Source: CAD feature listing. Evaluate the final solid. Frame: model axes, mm. A direction names the side the tool comes from. Give positions to 0.01 mm unless a question says otherwise; leave off trailing zeros. Write each loop counter-clockwise with the first axis right and the second up, starting at its lowest first coordinate (ties: lowest second). Pieces come first, ordered by that corner, then holes. Notation, with made-up numbers: (80.5, 61.25) -> (106.5, 61.25) arc R22 cw to (106.5, 84.25) -> close; hole circle Ø2 at (4, 88). An arc over 180 degrees is marked (long way). Use a Markdown table: item, result. Add a question column.
```python
from build123d import *

# Parameters (mm, degrees)
F0_W      = 51
F0_H      = 26
F1_DEPTH  = 1.5
F2_W      = 2
F2_H      = 2
F3_DEPTH  = 13
F5_DEPTH  = 13
F6_W      = 4
F6_H      = 2.5
F7_DEPTH  = 2.5
F8_R      = 0.75
F9_DEPTH  = 1.501
F11_DEPTH = 2
F12_W     = 8
F12_H     = 5
F13_DEPTH = 1.2


with BuildPart() as f1:
    # F0 (on Top) → F1 (new body)
    with BuildSketch(Plane.XY):
        Rectangle(F0_W, F0_H)
    extrude(amount=F1_DEPTH)

    # F2 (on face) → F3 (join)
    with BuildSketch(Plane.XY.offset(1.5)):
        with Locations((-24.5, 8.4)):
            Rectangle(F2_W, F2_H)
        Polygon((-19.5, 11.4), (-25.5, 11.4), (-25.5, 9.4), (-23.5, 9.4), (-21.5, 9.4), (-19.5, 9.4), align=None)
        with Locations((-20.5, 8.4)):
            Rectangle(F2_W, F2_H)
        with Locations((-24.5, -8.4)):
            Rectangle(F2_W, F2_H)
        Polygon((-23.5, -9.4), (-25.5, -9.4), (-25.5, -11.4), (-19.5, -11.4), (-19.5, -9.4), (-21.5, -9.4), align=None)
        with Locations((-20.5, -8.4)):
            Rectangle(F2_W, F2_H)
    extrude(amount=F3_DEPTH)

    # F4 (on face) → F5 (join)
    with BuildSketch(Plane.XY.offset(1.5)):
        Polygon((-19.5, 10.5), (-19.5, 9.15), (24.3, 9.15), (24.3, -9.15), (-19.5, -9.15), (-19.5, -10.5), (25.5, -10.5), (25.5, 10.5), align=None)
    extrude(amount=F5_DEPTH)

    # F6 (on face) → F7 (join)
    with BuildSketch(Plane.XY.offset(1.5)):
        Polygon((-15.5, 9.15), (-19.5, 9.15), (-19.5, 7.4), (-19.5, 6.65), (-15.5, 6.65), align=None)
        with Locations((22.3, 7.9)):
            Rectangle(F6_W, F6_H)
        with Locations((22.3, -7.9)):
            Rectangle(F6_W, F6_H)
        Polygon((-19.5, -9.15), (-15.5, -9.15), (-15.5, -6.65), (-19.5, -6.65), (-19.5, -7.4), align=None)
    extrude(amount=F7_DEPTH)

    # F8 (on face) → F9 (cut, through all)
    with BuildSketch(Plane.XY.offset(1.5)):
        with Locations((-18.5, 11.5)):
            Circle(F8_R)
        with Locations((2.5, 11.5)):
            Circle(F8_R)
        with Locations((23.5, 11.5)):
            Circle(F8_R)
        with Locations((-18.5, -11.5)):
            Circle(F8_R)
        with Locations((2.5, -11.5)):
            Circle(F8_R)
        with Locations((23.5, -11.5)):
            Circle(F8_R)
    extrude(amount=-F9_DEPTH, mode=Mode.SUBTRACT)

    # F10 (on face) → F11 (cut)
    with BuildSketch(Plane.XY.offset(1.5)):
        Polygon((-21.5, 9.4), (-23.5, 9.4), (-23.5, 7.4), (-23.5, -7.4), (-23.5, -9.4), (-21.5, -9.4), (-21.5, -7.4), (-21.5, 7.4), align=None)
    extrude(amount=-F11_DEPTH, mode=Mode.SUBTRACT)

    # F12 (on face) → F13 (cut, through all)
    with BuildSketch(Plane.YZ.offset(25.5)):
        with Locations((0, 7.5)):
            Rectangle(F12_W, F12_H)
    extrude(amount=-F13_DEPTH, mode=Mode.SUBTRACT)


solid = f1.part
```
(1) First-contact query: pin 1 Ø4 at (x, z) = (6, 11) entering from -Y; pin 2 Ø3 at (x, z) = (0, 7) entering from +Y; pin 3 Ø1.7 at (x, y) = (23.5, 11.5) entering from +Z. Flat tips, straight axial feed; report the tip coordinate or a pass-through.
(2) Cut plane B-B on x = -18.5. Return the cut outline in (y, z), then the cut area to 3 significant figures.
(3) Cut plane A-A on z = 5.75. Return the cut outline in (x, y).
(4) Access query for faces 1 (the flat face through (-19.5, -11, 8)), 2 (the flat face through (-15.5, 8, 3)), 3 (the flat face through (-23, -9.4, 7)), 4 (the flat face through (-21, 7.4, 8)), 5 (the flat face through (25, -4, 7)). Directions: +Z, -Z, +X, -X, +Y, -Y. A direction counts if a zero-diameter tool reaches every point of the face in a straight line with its end or side. Return the directions, or none.
(5) Cut plane D-D on z = 1. Return the cut outline in (x, y).
(6) Cut plane C-C on y = -4.5. Return the cut outline in (x, z).
(7) Material intervals for L1, parallel to Y at x = 23.5, z = 0.3; L2, parallel to X at y = -8.5, z = 5.75; L3, parallel to Y at x = -12.5, z = 12.75, sorted ascending.
(8) Mould query, pull axis Y, two halves, no side actions, for faces 6 (the flat face through (3, -9.15, 8)), 7 (the flat face through (3, -10.5, 8)), 8 (the flat face through (0, 0, 0)). Classes: +Y half, -Y half, draft (parallel to the pull), parting line (faces both ways), or undercut.
Output:
| question | item | result |
|---|---|---|
| 1 | pin 1 | y = -10.5 |
| 1 | pin 2 | y = 10.5 |
| 1 | pin 3 | z = 1.5 |
| 2 | outline | (-13, 0) -> (-12.25, 0) -> (-12.25, 1.5) -> (-13, 1.5) -> close; (-10.75, 0) -> (10.75, 0) -> (10.75, 1.5) -> (10.5, 1.5) -> (10.5, 14.5) -> (9.15, 14.5) -> (9.15, 4) -> (6.65, 4) -> (6.65, 1.5) -> (-6.65, 1.5) -> (-6.65, 4) -> (-9.15, 4) -> (-9.15, 14.5) -> (-10.5, 14.5) -> (-10.5, 1.5) -> (-10.75, 1.5) -> close; (12.25, 0) -> (13, 0) -> (13, 1.5) -> (12.25, 1.5) -> close |
| 2 | area | 82.1 mm^2 |
| 3 | outline | (-25.5, -11.4) -> (-19.5, -11.4) -> (-19.5, -10.5) -> (25.5, -10.5) -> (25.5, -4) -> (24.3, -4) -> (24.3, -9.15) -> (-19.5, -9.15) -> (-19.5, -7.4) -> (-21.5, -7.4) -> (-21.5, -9.4) -> (-23.5, -9.4) -> (-23.5, -7.4) -> (-25.5, -7.4) -> close; (-25.5, 7.4) -> (-23.5, 7.4) -> (-23.5, 9.4) -> (-21.5, 9.4) -> (-21.5, 7.4) -> (-19.5, 7.4) -> (-19.5, 9.15) -> (24.3, 9.15) -> (24.3, 4) -> (25.5, 4) -> (25.5, 10.5) -> (-19.5, 10.5) -> (-19.5, 11.4) -> (-25.5, 11.4) -> close |
| 4 | face 1 | +Z, +X, -Y |
| 4 | face 2 | +Z |
| 4 | face 3 | +Z, -Z |
| 4 | face 4 | +Z, -X |
| 4 | face 5 | +X, -X |
| 5 | outline | (-25.5, -13) -> (25.5, -13) -> (25.5, 13) -> (-25.5, 13) -> close; hole (-23.5, -9.4) -> (-21.5, -9.4) -> (-21.5, 9.4) -> (-23.5, 9.4) -> close; hole circle Ø1.5 at (-18.5, -11.5); hole circle Ø1.5 at (-18.5, 11.5); hole circle Ø1.5 at (2.5, -11.5); hole circle Ø1.5 at (2.5, 11.5); hole circle Ø1.5 at (23.5, -11.5); hole circle Ø1.5 at (23.5, 11.5) |
| 6 | outline | (-25.5, 0) -> (-23.5, 0) -> (-23.5, 1.5) -> (-25.5, 1.5) -> close; (-21.5, 0) -> (25.5, 0) -> (25.5, 14.5) -> (24.3, 14.5) -> (24.3, 1.5) -> (-21.5, 1.5) -> close |
| 7 | L1 | -13 to -12.25, -10.75 to 10.75, 12.25 to 13 |
| 7 | L2 | -25.5 to -23.5, -21.5 to -19.5, 24.3 to 25.5 |
| 7 | L3 | -10.5 to -9.15, 9.15 to 10.5 |
| 8 | face 6 | undercut |
| 8 | face 7 | -Y half |
| 8 | face 8 | draft |
